Verification items for the finished model (mm, model axes). Coordinates: 2 decimals unless noted, no trailing zeros. Order: outer loops, then holes, each group sorted by start corner. A loop starts at its lowest first (then second) coordinate and runs counter-clockwise, first axis right, second up. Notation, with made-up numbers: (-23.5, -33.5) -> (8.5, -33.5) arc R11 ccw to (8.5, -15.5) -> close; hole circle Ø5 at (70.25, -16.75). An arc over 180 degrees is marked (long way). Answer as CSV lines item,"result".
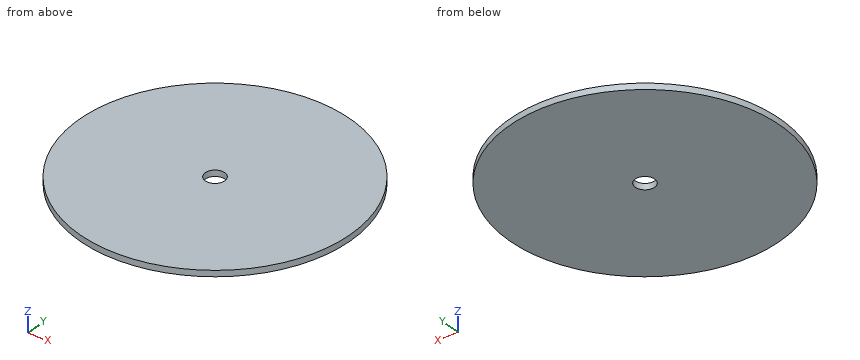
```python
from build123d import *

# Parameters (mm, degrees)
F0_R     = 57.15
F1_DEPTH = 2.54
F2_R     = 4.09365
F3_DEPTH = 25.4
F4_DEPTH = 25.4


with BuildPart() as f1:
    # F0 (on Top) → F1 (new body)
    with BuildSketch(Plane.XY):
        Circle(F0_R)
    extrude(amount=F1_DEPTH)

    # F2 (on Top) → F3 (cut)
    with BuildSketch(Plane.XY):
        Circle(F2_R)
    extrude(amount=-F3_DEPTH, mode=Mode.SUBTRACT)

    # F2 (on Top) → F4 (cut)
    with BuildSketch(Plane.XY):
        Circle(F2_R)
    extrude(amount=F4_DEPTH, mode=Mode.SUBTRACT)


solid = f1.part
```
Item 1: Depth check by flat-ended pin: pin 1 Ø1.5 at (x, z) = (-32.5, 0.5) entering from +Y. Enter the tip coordinate at first touch or a pass-through.
Answer list:
pin 1,"y = 47.52"
Item 2: Thickness scan on line 1 (Y direction, x = 0, z = 1.25); line 2 (Y direction, x = -29.5, z = 2); line 3 (X direction, y = -30.5, z = 2.45). Record the ranges inside material, lowest first.
Answer list:
line 1,"-57.15 to -4.09, 4.09 to 57.15"
line 2,"-48.95 to 48.95"
line 3,"-48.33 to 48.33"
Item 3: Section check C-C, the plane z = 0.65. Record the boundary of the cut face in (x, y).
Answer list:
outline,"circle Ø114.3 at (0, 0); hole circle Ø8.19 at (0, 0)"
Item 4: Section check D-D, the plane x = 13.5. Record the boundary of the cut face in (y, z).
Answer list:
outline,"(-55.53, 0) -> (55.53, 0) -> (55.53, 2.54) -> (-55.53, 2.54) -> close"
Item 5: Section check A-A, the plane y = 0. Record the boundary of the cut face in (x, z), plus the area to 3 significant figures.
Answer list:
outline,"(-57.15, 0) -> (-4.09, 0) -> (-4.09, 2.54) -> (-57.15, 2.54) -> close; (4.09, 0) -> (57.15, 0) -> (57.15, 2.54) -> (4.09, 2.54) -> close"
area,"270 mm2"
